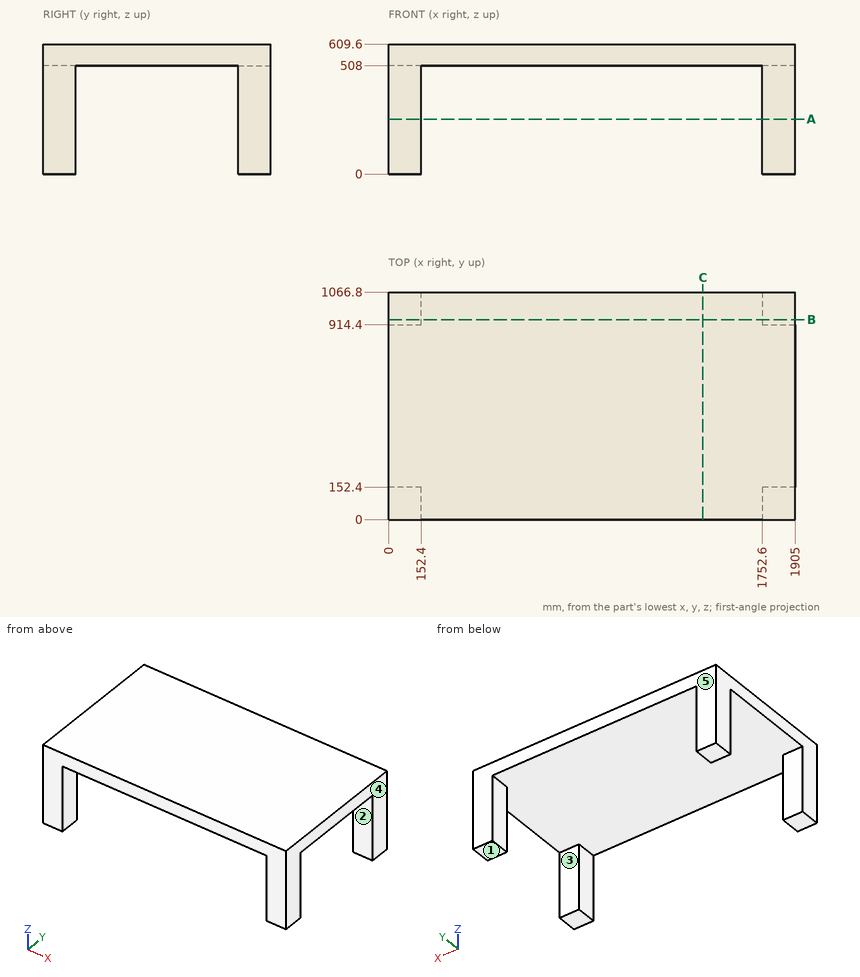
Check sheet for the drawn part. Datum: minimum x, y, z corner. Units: mm. A direction names the side the tool comes from. Round coordinates to 2 decimals unless told otherwise and drop trailing zeros. Write each loop counter-clockwise with the first axis right and the second up, starting at its lowest first coordinate (ties: lowest second). Pieces come first, ordered by that corner, then holes. Notation, with made-up numbers: (-1, 6) -> (38, 6) arc R26 cw to (38, 30) -> close; hole circle Ø9 at (20.5, 83). An arc over 180 degrees is marked (long way). Write each question's results on one line, items separated by ' | '. Start each with the question number.
1. Draft check along Y on the marked faces 3, 4 and 5. Enter one of: +Y half, -Y half, draft (parallel to the pull), parting line (faces both ways), or undercut.
2. Set-up check for the marked faces 1 and 2: record each of +Z, -Z, +X, -X, +Y, -Y from which the full face is reachable in a straight line by a thin tool's end or side.
3. Material ranges on probe 1 along Y at (x, z) = (1825.5, 190); probe 2 along X at (y, z) = (957.5, 273.5); probe 3 along Z at (x, y) = (1628.5, 222), recorded low to high. Write a range as from..to.
4. Cross-section at C-C (x = 1473). Enter the section's corners in (y, z).
5. Cross-section at B-B (y = 937). Enter the section's corners in (x, z).
6. Cross-section at A-A (z = 257). Enter the section's corners in (x, y), then the cut area to 3 significant figures.
Solutions:
1) face 3: undercut | face 4: draft | face 5: +Y half
2) face 1: -Z, +X, -X, +Y, -Y | face 2: -Z, +X, -X
3) probe 1: y = 0..152.4, 914.4..1066.8 | probe 2: x = 0..152.4, 1752.6..1905 | probe 3: z = 508..609.6
4) outline: (0, 508) -> (1066.8, 508) -> (1066.8, 609.6) -> (0, 609.6) -> close
5) outline: (0, 0) -> (152.4, 0) -> (152.4, 508) -> (1752.6, 508) -> (1752.6, 0) -> (1905, 0) -> (1905, 609.6) -> (0, 609.6) -> close
6) outline: (0, 0) -> (152.4, 0) -> (152.4, 152.4) -> (0, 152.4) -> close; (0, 914.4) -> (152.4, 914.4) -> (152.4, 1066.8) -> (0, 1066.8) -> close; (1752.6, 0) -> (1905, 0) -> (1905, 152.4) -> (1752.6, 152.4) -> close; (1752.6, 914.4) -> (1905, 914.4) -> (1905, 1066.8) -> (1752.6, 1066.8) -> close | area: 92,900 mm2
